Geometry check sheet. Reference: the model listing, model coordinates, mm. Face numbers are marked on the shaded views. Round coordinates to 2 decimals unless told otherwise and drop trailing zeros. Write each loop counter-clockwise with the first axis right and the second up, starting at its lowest first coordinate (ties: lowest second). Pieces come first, ordered by that corner, then holes. Notation, with made-up numbers: M -18.5,9 L 25.5,9 A34 cw 25.5,41 Z; hole C 60,23 d7. An arc over 180 degrees is marked long. Answer in a Markdown table with one row per item. Add a question column.
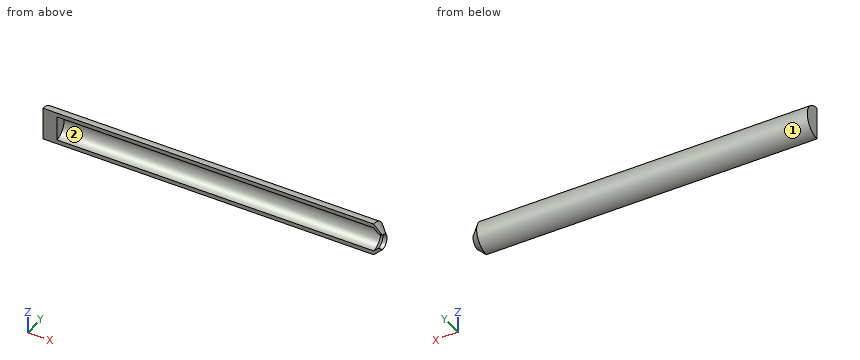
from build123d import *

# Parameters (mm, degrees)
BOSS_EXTRUDE1_DEPTH = 60
BOSS_EXTRUDE2_START = -5
BOSS_EXTRUDE2_DEPTH = 5
REVOLVE1_ANGLE      = 180


with BuildPart() as part:
    # Sketch1 → Boss-Extrude1 (new, symmetric)
    with BuildSketch(Plane(origin=(0, 0, 0), x_dir=(0, 0, -1), z_dir=(1, 0, 0))):
        with BuildLine():
            Line((-6, 0), (-4.5, 0))
            ThreePointArc((-4.5, 0), (0, 4.5), (4.5, 0))
            Line((4.5, 0), (6, 0))
            ThreePointArc((6, 0), (0, 6), (-6, 0))
        make_face()
    extrude(amount=BOSS_EXTRUDE1_DEPTH, both=True)

    # Sketch2 → Boss-Extrude2 (add)
    with BuildSketch(Plane.ZY.offset(60).offset(BOSS_EXTRUDE2_START)):
        with BuildLine():
            Line((-4.5, 0), (4.5, 0))
            ThreePointArc((4.5, 0), (0, 4.5), (-4.5, 0))
        make_face()
    extrude(amount=BOSS_EXTRUDE2_DEPTH)

    # Sketch3 → Revolve1 (revolve)
    with BuildSketch(Plane.XZ):
        Polygon((60, 6), (63.2, 2.8), (61.7, 2.8), (60, 4.5), align=None)
    revolve(axis=Axis((0, 0, 0), (-1, 0, 0)), revolution_arc=REVOLVE1_ANGLE)


solid = part.part
Item 1: Gauge pin test, flat ends, axial feed: pin 1 Ø1 at (x, y) = (-9, 5.5) entering from +Z; pin 2 Ø4 at (x, z) = (-33, 0.5) entering from -Y. Record the tip position at first contact, or that the pin passes through.
Item 2: Scan lines: probe 1 along Z at (x, y) = (50.5, 0.6); probe 2 along X at (y, z) = (4.15, -1); probe 3 along Y at (x, z) = (-21, 0). Record each from-to range of solid material in increasing order. Write a range as from..to.
Item 3: Section check A-A, the plane z = 0. Record the boundary of the cut face in (x, y), and give its area (3 significant figures).
Item 4: Section check B-B, the plane x = -38.5. Record the boundary of the cut face in (y, z).
Item 5: Mould release check, pull along Z, two halves, no side actions. Record for the marked faces 1 and 2: +Z half, -Z half, draft (parallel to the pull), parting line (faces both ways), or undercut.
Result sheet:
| question | item | result |
|---|---|---|
| 1 | pin 1 | stops at z = 3.32 |
| 1 | pin 2 | stops at y = 3.74 |
| 2 | probe 1 | z = -5.97..-4.46, 4.46..5.97 |
| 2 | probe 2 | x = -60..-55, 60.23..61.73 |
| 2 | probe 3 | y = 4.5..6 |
| 3 | outline | M -60,0 L -55,0 L -55,4.5 L 60,4.5 L 61.7,2.8 L 63.2,2.8 L 60,6 L -60,6 Z |
| 3 | area | 206 mm^2 |
| 4 | outline | M 0,-6 A6 ccw 0,6 L 0,4.5 A4.5 cw 0,-4.5 Z |
| 5 | face 1 | parting line |
| 5 | face 2 | undercut |
